For this review, use the dimensioned drawing (mm, ordinates from the lowest corner) and the shaded views. A direction names the side the tool comes from. Round coordinates to 2 decimals unless told otherwise and drop trailing zeros. Loops run counter-clockwise (first coordinate to the right, second up) from the corner with the lowest first, then second, coordinate; pieces in that order, holes last. Notation, with made-up numbers: (-5.5, -11) - (16.5, -11) arc R33 ccw to (16.5, 28) - close; hole circle Ø5 at (25, -16.5). An arc over 180 degrees is marked (long way). Return JSON: item names as keys, results as strings. Group by question number.
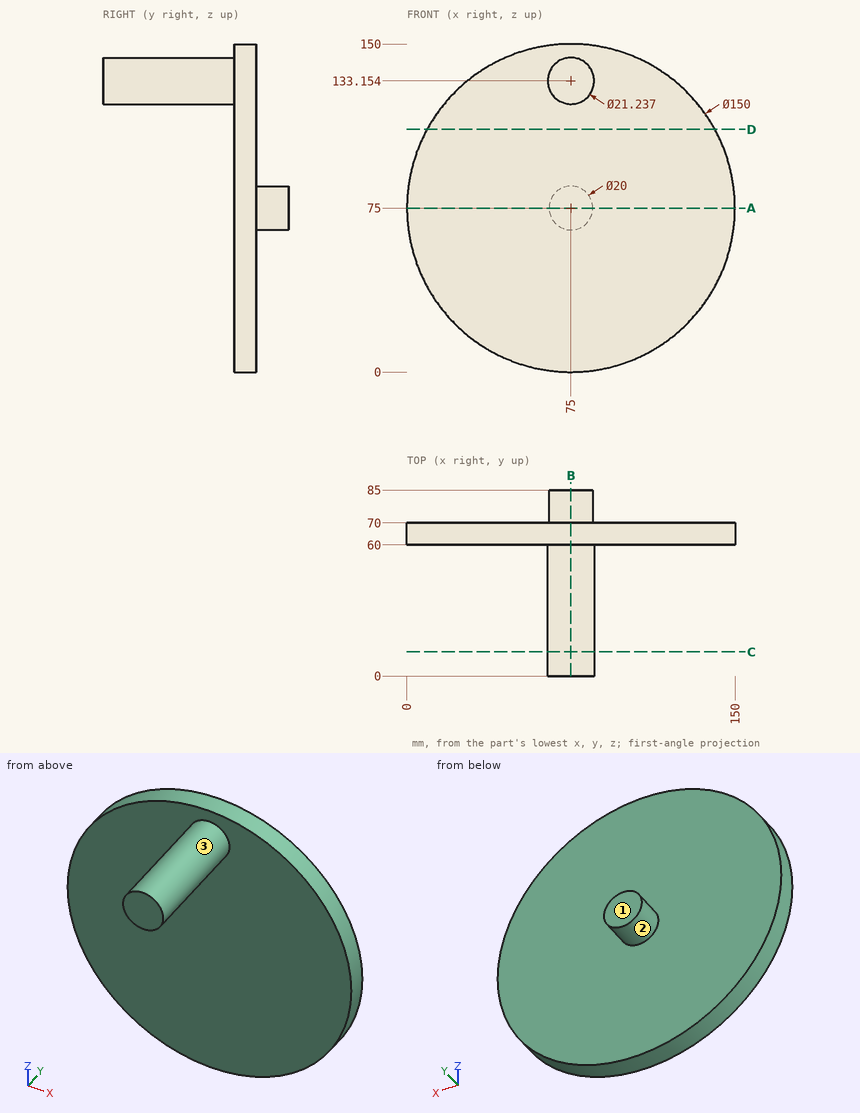
Q1. Add section A-A, the plane z = 75. State the section outline as (x, y) points.
Q2. Add section C-C, the plane y = 11. State the section outline as (x, z) points.
Q3. Add section B-B, the plane x = 75. State the section outline as (y, z) points (1 decimal).
Q4. Insertion check: pin 1 Ø2 at (x, y) = (68.5, 49.5) entering from -Z; pin 2 Ø10 at (x, z) = (108, 81.5) entering from -Y; pin 3 Ø3 at (x, y) = (17.5, 59) entering from +Z. Each pin has a flat end and moves straight along its axis. Give the tip position at first contact, or say it passes through.
Q5. For line 1 (Y direction, x = 19, z = 71); line 2 (X direction, y = 27, z = 133.5); line 3 (X direction, y = 61.5, z = 126.5) (1 decimal), list the stretches that pass through material, from the lowest coordinate up.
Q6. Tool access review of the marked faces 1, 2 and 3: name each direction out of +Z, -Z, +X, -X, +Y, -Y from which nothing blocks a thin tool from reaching the whole face with its end or side.
Q7. Add section D-D, the plane z = 111. State the section outline as (x, y) points (1 decimal), plus the area to 3 significant figures.
Evaluation:
{
 "1": {"outline": "(0, 60) - (150, 60) - (150, 70) - (85, 70) - (85, 85) - (65, 85) - (65, 70) - (0, 70) - close"},
 "2": {"outline": "circle Ø21.24 at (75, 133.15)"},
 "3": {"outline": "(0, 122.5) - (60, 122.5) - (60, 0) - (70, 0) - (70, 65) - (85, 65) - (85, 85) - (70, 85) - (70, 150) - (60, 150) - (60, 143.8) - (0, 143.8) - close"},
 "4": {"pin 1": "z = 124.07", "pin 2": "y = 60", "pin 3": "z = 124.46"},
 "5": {"line 1": "60 to 70", "line 2": "64.39 to 85.61", "line 3": "20.5 to 129.5"},
 "6": {"face 1": "+Z, -Z, +X, -X, +Y", "face 2": "+Y", "face 3": "-Y"},
 "7": {"outline": "(9.2, 60) - (140.8, 60) - (140.8, 70) - (9.2, 70) - close", "area": "1,320 mm²"}
}
